Autodesk Inventor part; units mm, degrees
ref_plane "YZ Plane" through (0, 0, 0) normal (1, 0, 0) x (0, 1, 0)
ref_plane "XZ Plane" through (0, 0, 0) normal (0, 1, 0) x (-1, 0, 0)
ref_plane "XY Plane" through (0, 0, 0) normal (0, 0, 1) x (1, 0, 0)
sketch "Sketch1" plane through (0, 0, 0) normal (0, 1, 0) x (-1, 0, 0)
  line L0 (0, 0) -> (-80.01, 0)
  line L1 (-80.01, 0) -> (-80.01, -80.01)
  line L2 (-80.01, -80.01) -> (0, -80.01)
  line L3 (0, -80.01) -> (0, 0)
  dimension "d0" = 80.01
  dimension "d1" = 80.01
extrude "Extrusion1" add sketch "Sketch1" along normal blind 1.524
sketch "Sketch2" plane through (0, 1.524, 0) normal (0, 1, 0) x (1, 0, 0)
  line L0 (0, 0) -> (80.01, 0)
  line L1 (80.01, 80.01) -> (0, 80.01)
  line L2 (0, 0) -> (8.001, 0)
  line L3 (8.001, 0) -> (8.001, 8.001)
  circle A0 centre (8.001, 8.001) radius 1.5
  line L4 (80.01, 0) -> (72.009, 0)
  line L5 (72.009, 0) -> (72.009, 8.001)
  line L6 (0, 80.01) -> (8.001, 80.01)
  line L7 (8.001, 80.01) -> (8.001, 72.009)
  line L8 (80.01, 80.01) -> (72.009, 80.01)
  line L9 (72.009, 80.01) -> (72.009, 72.009)
  circle A1 centre (8.001, 72.009) radius 1.4986
  circle A2 centre (72.009, 72.009) radius 1.4986
  circle A3 centre (72.009, 8.001) radius 1.4986
  line L10 (0, 0) -> (15.0114, 0)
  line L11 (15.0114, 0) -> (15.0114, 15.0114)
  line L12 (0, 80.01) -> (15.0114, 80.01)
  line L13 (15.0114, 80.01) -> (15.0114, 64.9986)
  line L14 (80.01, 80.01) -> (64.9986, 80.01)
  line L15 (64.9986, 80.01) -> (64.9986, 64.9986)
  line L16 (80.01, 0) -> (64.9986, 0)
  line L17 (64.9986, 0) -> (64.9986, 15.0114)
  circle A4 centre (15.0114, 15.0114) radius 1.4986
  circle A5 centre (15.0114, 64.9986) radius 1.4986
  circle A6 centre (64.9986, 64.9986) radius 1.4986
  circle A7 centre (64.9986, 15.0114) radius 1.4986
  dimension "d4" = 8.001
  dimension "d5" = 8.001
  dimension "d6" = 3
  dimension "d7" = 8.001
  dimension "d8" = 8.001
  dimension "d9" = 8.001
  dimension "d10" = 8.001
  dimension "d11" = 8.001
  dimension "d12" = 2.9972
  dimension "d13" = 2.9972
  dimension "d14" = 15.0114
  dimension "d15" = 15.0114
  dimension "d16" = 15.0114
  dimension "d17" = 15.0114
  dimension "d18" = 15.0114
  dimension "d19" = 15.0114
  dimension "d20" = 15.0114
  dimension "d21" = 15.0114
  dimension "d22" = 2.9972
  dimension "d23" = 2.9972
  dimension "d24" = 2.9972
  dimension "d25" = 2.9972
extrude "Extrusion2" cut sketch "Sketch2" against normal blind 1.524
sketch "Sketch3" plane through (0, 1.524, 0) normal (0, 1, 0) x (1, 0, 0)
  line L0 (0, 0) -> (80.01, 0)
  line L1 (80.01, 0) -> (80.01, 80.01)
  line L2 (80.01, 80.01) -> (0, 80.01)
  line L3 (0, 80.01) -> (0, 0)
  line L4 (40.005, 0) -> (40.005, 7.62)
  line L5 (0, 40.005) -> (7.62, 40.005)
  line L6 (40.005, 80.01) -> (40.005, 72.39)
  line L7 (80.01, 40.005) -> (72.39, 40.005)
  circle A0 centre (40.005, 72.39) radius 4.445
  circle A1 centre (40.005, 7.62) radius 4.445
  circle A2 centre (7.62, 40.005) radius 4.445
  circle A3 centre (72.39, 40.005) radius 4.445
  circle A4 centre (7.62, 28.575) radius 4.445
  circle A5 centre (72.39, 28.575) radius 4.445
  circle A6 centre (7.62, 51.435) radius 4.445
  circle A7 centre (72.39, 51.435) radius 4.445
  circle A8 centre (7.62, 40.005) radius 4.445
  circle A9 centre (72.39, 40.005) radius 4.445
  circle A10 centre (51.435, 72.39) radius 4.445
  circle A11 centre (51.435, 7.62) radius 4.445
  circle A12 centre (28.575, 72.39) radius 4.445
  circle A13 centre (28.575, 7.62) radius 4.445
  circle A14 centre (40.005, 72.39) radius 4.445
  circle A15 centre (40.005, 7.62) radius 4.445
  line L8 (19.05, 40.005) -> (19.05, 45.72)
  line L9 (19.05, 40.005) -> (19.05, 34.29)
  circle A16 centre (19.05, 45.72) radius 4.445
  circle A17 centre (19.05, 34.29) radius 4.445
  line L10 (7.62, 40.005) -> (19.05, 40.005)
  line L11 (19.05, 40.005) -> (30.48, 40.005)
  circle A18 centre (30.48, 40.005) radius 4.445
  line L12 (40.005, 72.39) -> (40.005, 60.96)
  line L13 (40.005, 60.96) -> (40.005, 49.53)
  line L14 (72.39, 40.005) -> (60.96, 40.005)
  line L15 (60.96, 40.005) -> (49.53, 40.005)
  line L16 (40.005, 7.62) -> (40.005, 19.05)
  line L17 (40.005, 19.05) -> (40.005, 30.48)
  line L18 (40.005, 19.05) -> (45.72, 19.05)
  line L19 (40.005, 19.05) -> (34.29, 19.05)
  line L20 (40.005, 60.96) -> (45.72, 60.96)
  line L21 (40.005, 60.96) -> (34.29, 60.96)
  line L22 (60.96, 40.005) -> (60.96, 45.72)
  line L23 (60.96, 40.005) -> (60.96, 34.29)
  circle A19 centre (40.005, 49.53) radius 4.445
  circle A20 centre (40.005, 30.48) radius 4.445
  circle A21 centre (49.53, 40.005) radius 4.445
  circle A22 centre (60.96, 45.72) radius 4.445
  circle A23 centre (60.96, 34.29) radius 4.445
  circle A24 centre (34.29, 60.96) radius 4.445
  circle A25 centre (45.72, 60.96) radius 4.445
  circle A26 centre (34.29, 19.05) radius 4.445
  circle A27 centre (45.72, 19.05) radius 4.445
  dimension "d28" = 7.62
  dimension "d29" = 7.62
  dimension "d30" = 7.62
  dimension "d31" = 7.62
  dimension "d32" = 8.89
  dimension "d33" = 8.89
  dimension "d34" = 8.89
  dimension "d35" = 8.89
  dimension "d45" = 11.43
  dimension "d52" = 11.43
  dimension "d66" = 11.43
  dimension "d69" = 11.43
  dimension "d74" = 11.43
  dimension "d77" = 11.43
  dimension "d111" = 5.715
  dimension "d112" = 5.715
  dimension "d113" = 8.89
  dimension "d114" = 8.89
  dimension "d115" = 11.43
  dimension "d116" = 8.89
  dimension "d117" = 11.43
  dimension "d118" = 11.43
  dimension "d119" = 11.43
  dimension "d120" = 11.43
  dimension "d121" = 11.43
  dimension "d122" = 5.715
  dimension "d123" = 5.715
  dimension "d124" = 5.715
  dimension "d125" = 5.715
  dimension "d126" = 5.715
  dimension "d127" = 5.715
  dimension "d128" = 8.89
  dimension "d129" = 8.89
  dimension "d130" = 8.89
  dimension "d131" = 8.89
  dimension "d132" = 8.89
  dimension "d133" = 8.89
  dimension "d134" = 8.89
  dimension "d135" = 8.89
  dimension "d136" = 8.89
sketch "Sketch4" plane through (0, 1.524, 0) normal (0, 1, 0) x (1, 0, 0)
  line L0 (0, 0) -> (80.01, 0)
  line L1 (0, 0) -> (24.7396, 0)
  line L2 (24.7396, 0) -> (24.7396, 24.7396)
  circle A0 centre (24.7396, 24.7396) radius 1.4986
  line L3 (80.01, 0) -> (55.2704, 0)
  line L4 (55.2704, 0) -> (55.2704, 24.7396)
  circle A1 centre (55.2704, 24.7396) radius 1.4986
  line L5 (80.01, 80.01) -> (0, 80.01)
  line L6 (0, 80.01) -> (24.7396, 80.01)
  line L7 (24.7396, 80.01) -> (24.7396, 55.2704)
  circle A2 centre (24.7396, 55.2704) radius 1.4986
  line L8 (80.01, 80.01) -> (55.2704, 80.01)
  line L9 (55.2704, 80.01) -> (55.2704, 55.2704)
  circle A3 centre (55.2704, 55.2704) radius 1.4986
  dimension "d98" = 24.7396
  dimension "d99" = 24.7396
  dimension "d100" = 2.9972
  dimension "d101" = 24.7396
  dimension "d102" = 24.7396
  dimension "d103" = 2.9972
  dimension "d104" = 24.7396
  dimension "d105" = 24.7396
  dimension "d106" = 2.9972
  dimension "d107" = 24.7396
  dimension "d108" = 24.7396
extrude "Extrusion4" cut sketch "Sketch4" against normal blind 25.4
extrude "Extrusion5" cut sketch "Sketch3" against normal blind 25.4 contours A26 | A20 | A27 | A1 L16 L4 | L4 L16 A1 | A23 | A21 | A22 | A3 L14 L7 | L7 L14 A3 | A25 | A19 | A24 | A0 L12 L6 | L6 L12 A0 | A16 | A18 | A17 | A2 L10 L5 | L5 L10 A2 | A4 | A5 | A6 | A7 | A10 | A11 | A12 | A13
properties part number "plate_mk2"
Source: CAD feature listing. Evaluate the final solid. Frame: model axes, mm. Give positions to 0.01 mm unless a question says otherwise; leave off trailing zeros. Write each loop counter-clockwise with the first axis right and the second up, starting at its lowest first coordinate (ties: lowest second). Pieces come first, ordered by that corner, then holes. Notation, with made-up numbers: M 29.25,45 L 74.25,45 A33 cw 74.25,81 Z; hole C 36.25,16 d8. An arc over 180 degrees is marked long. Return JSON: item names as keys, results as strings. Group by question number.
1) Pull-direction query (X, two-part tool) for faces 1 (the face through (7.04, 0.77, -44.41)), 2 (the face through (65.69, 0.77, -63.67)); classes: pulls with the +X half, pulls with the -X half, needs draft (parallel to the pull), parting line crosses it, or undercut.
2) Cut plane B-B, the plane x = 19.05. Output: boundary loops of the cut face in (y, z) (3 decimals), plus the area to 3 significant figures.
3) Material intervals for line 1 along X through (y, z) = (0.5, -40) (3 decimals); line 2 along X through (y, z) = (0.8, -60.96) (3 decimals); line 3 along X through (y, z) = (0.3, -23), sorted ascending. Write a range as [from, to].
4) Cut plane C-C, the plane z = -43. Output: boundary loops of the cut face in (x, y).
5) Cut plane A-A, the plane z = -60.96. Output: boundary loops of the cut face in (x, y) (3 decimals), plus the area to 3 significant figures.
6) Cut plane D-D, the plane x = 28. Output: boundary loops of the cut face in (y, z), plus the area to 3 significant figures.
7) Pin query (flat end, axial travel): P1, Ø8, axis at x = 24.5, z = -9, coming from the +Y side. Return the tip coordinate at first contact, or that it passes through.
Recorded:
{
 "1": {"face 1": "undercut", "face 2": "undercut"},
 "2": {"outline": "M 0,-80.01 L 1.524,-80.01 L 1.524,-50.165 L 0,-50.165 Z; M 0,-41.275 L 1.524,-41.275 L 1.524,-38.735 L 0,-38.735 Z; M 0,-29.845 L 1.524,-29.845 L 1.524,0 L 0,0 Z", "area": "94.8 mm²"},
 "3": {"line 1": "x = [0, 3.175], [12.065, 26.035], [34.925, 45.085], [53.975, 67.945], [76.835, 80.01]", "line 2": "x = [0, 29.845], [38.735, 41.275], [50.165, 80.01]", "line 3": "x = [0, 32.25], [36.33, 43.68], [47.76, 80.01]"},
 "4": {"outline": "M 0,0 L 4.34,0 L 4.34,1.52 L 0,1.52 Z; M 10.9,0 L 15.53,0 L 15.53,1.52 L 10.9,1.52 Z; M 22.57,0 L 27.2,0 L 27.2,1.52 L 22.57,1.52 Z; M 33.76,0 L 46.25,0 L 46.25,1.52 L 33.76,1.52 Z; M 52.81,0 L 57.44,0 L 57.44,1.52 L 52.81,1.52 Z; M 64.48,0 L 69.11,0 L 69.11,1.52 L 64.48,1.52 Z; M 75.67,0 L 80.01,0 L 80.01,1.52 L 75.67,1.52 Z"},
 "5": {"outline": "M 0,0 L 29.845,0 L 29.845,1.524 L 0,1.524 Z; M 38.735,0 L 41.275,0 L 41.275,1.524 L 38.735,1.524 Z; M 50.165,0 L 80.01,0 L 80.01,1.524 L 50.165,1.524 Z", "area": "94.8 mm²"},
 "6": {"outline": "M 0,-80.01 L 1.52,-80.01 L 1.52,-76.8 L 0,-76.8 Z; M 0,-67.98 L 1.52,-67.98 L 1.52,-43.69 L 0,-43.69 Z; M 0,-36.32 L 1.52,-36.32 L 1.52,-12.03 L 0,-12.03 Z; M 0,-3.21 L 1.52,-3.21 L 1.52,0 L 0,0 Z", "area": "83.8 mm²"},
 "7": {"P1": "stops at y = 1.52"}
}
